Design review of the part built by this model. Coordinates are the model's own, in mm. A direction names the side the tool comes from. Coordinates: 2 decimals unless noted, no trailing zeros. Loops run counter-clockwise (first coordinate to the right, second up) from the corner with the lowest first, then second, coordinate; pieces in that order, holes last. Notation, with made-up numbers: M 64.25,-5 L 108.25,-5 A32 ccw 108.25,30 Z; hole C -30,55.5 d11. An arc over 180 degrees is marked long. Answer as a JSON object with one key per item and string values. Group by question number.
1. Consider section C-C (x = 4.4). State the section outline as (y, z) points, then the cut area to 3 significant figures.
2. Draft analysis for pull direction Y (two halves, no side actions). For faces 4 (the flat face through (6, 8, -8)), 5 (the cylindrical face through (5.778, -2.341, -10.543)), 6 (the cylindrical face through (2.96, -11.99, -0.53)), 7 (the cylindrical face through (0.22, -5.75, -5.27)), state which applies: +Y half, -Y half, draft (parallel to the pull), parting line (faces both ways), or undercut.
3. Insertion check: pin 1 (1 mm diameter, centred on x = 2, y = 5, fed in from +Z); pin 2 (11 mm diameter, centred on y = 0, z = 0, fed in from -X); pin 3 (2 mm diameter, centred on x = 1.5, z = -9.5, fed in from +Y). Each pin has a flat end and moves straight along its axis. Give the tip position at first contact, or say it passes through.
4. To check wall thickness, follow probe 1 along Z at (x, y) = (5.75, 0); probe 2 along Z at (x, y) = (2.6, 0); probe 3 along X at (y, z) = (-6.5, 5.75). State the ranges of each line that lie inside material, in increasing order.
5. Machinability: for faces 1 (the flat face through (0, 8, -8)), 2 (the cylindrical face through (0.228, -2.341, -10.543)), 3 (the cylindrical face through (5.77, -5.75, -5.27)), which of the approach directions +Z, -Z, +X, -X, +Y, -Y give a long, thin tool a straight path to every point of the face, cutting with its end or side? Answer none if there is none.
Autodesk Inventor part; units mm, degrees
ref_plane "center_point_XY" through (3, 0, 0) normal (1, 0, 0) x (0, 0, -1)
ref_plane "center_point_YZ" through (3, 0, 0) normal (0, 0, -1) x (0, 1, 0)
ref_plane "center_point_ZX" through (3, 0, 0) normal (0, 1, 0) x (1, 0, 0)
sketch "Sketch_1" plane through (0, 0, 0) normal (0, 0, 1) x (1, 0, 0)
  line L0 (6, 0) -> (0, 0)
  arc A0 (0, 6.3) -> (0.3, 6) centre (0.3, 6.3) ccw
  line L1 (0.3, 6) -> (5.7, 6)
  arc A1 (5.7, 6) -> (6, 6.3) centre (5.7, 6.3) ccw
  line L2 (6, 6.3) -> (6, 7.8)
  line L3 (6, 7.8) -> (5.55, 7.8)
  line L4 (5.55, 7.8) -> (5.55, 10.8)
  line L5 (5.55, 10.8) -> (6, 10.8)
  line L6 (6, 10.8) -> (6, 11.7)
  arc A2 (6, 11.7) -> (5.7, 12) centre (5.7, 11.7) ccw
  line L7 (5.7, 12) -> (0.3, 12)
  arc A3 (0.3, 12) -> (0, 11.7) centre (0.3, 11.7) ccw
  line L8 (0, 11.7) -> (0, 10.8)
  line L9 (0, 10.8) -> (0.45, 10.8)
  line L10 (0.45, 10.8) -> (0.45, 7.8)
  line L11 (0.45, 7.8) -> (0, 7.8)
  line L12 (0, 7.8) -> (0, 6.3)
revolve "Revolution1" add sketch "Sketch_1" angle 360 about axis through (6, 0, 0) along (1, 0, 0)
ref_plane "center_point_XY" through (3, 0, 0) normal (1, 0, 0) x (0, 0, -1)
ref_plane "center_point_YZ" through (3, 0, 0) normal (0, 0, -1) x (0, 1, 0)
ref_plane "center_point_ZX" through (3, 0, 0) normal (0, 1, 0) x (1, 0, 0)
ref_plane "to_housing_XY" through (0, 0, 0) normal (1, 0, 0) x (0, 0, -1)
ref_plane "to_housing_YZ" through (0, 0, 0) normal (0, 0, -1) x (0, 1, 0)
ref_plane "to_housing_ZX" through (0, 0, 0) normal (0, 1, 0) x (1, 0, 0)
ref_plane "to_ring_XY" through (5.1, 0, 0) normal (1, 0, 0) x (0, 0, -1)
ref_plane "to_ring_YZ" through (5.1, 0, 0) normal (0, 0, -1) x (0, 1, 0)
ref_plane "to_ring_ZX" through (5.1, 0, 0) normal (0, 1, 0) x (1, 0, 0)
properties part number "B6901ZZ" material "鋼、炭素鋼"
Findings below:
{
 "1": {"outline": "C 0,0 d24; hole C 0,0 d12", "area": "339 mm^2"},
 "2": {"face 4": "draft", "face 5": "undercut", "face 6": "parting line", "face 7": "undercut"},
 "3": {"pin 1": "stops at z = 11.12", "pin 2": "passes through", "pin 3": "stops at y = 8.47"},
 "4": {"probe 1": "z = -12 to -10.8, -7.8 to -6, 6 to 7.8, 10.8 to 12", "probe 2": "z = -12 to -6, 6 to 12", "probe 3": "x = 0.45 to 5.55"},
 "5": {"face 1": "+Z, -Z, -X, +Y, -Y", "face 2": "-X", "face 3": "+X"}
}
